Could you check a few things on this model? Use its own coordinates, in mm. A direction names the side the tool comes from. Coordinates: 2 decimals unless noted, no trailing zeros. Loops run counter-clockwise (first coordinate to the right, second up) from the corner with the lowest first, then second, coordinate; pieces in that order, holes last. Notation, with made-up numbers: M -37,31.25 L 2,31.25 A23 ccw 2,66.25 Z; hole C -9.5,32 d4. An arc over 180 degrees is marked long. Write each question's results on one line, items separated by ' | '.
Autodesk Fusion 360 part; units mm, degrees
sketch "Sketch1" plane through (0, 0, 0) normal (1, 0, 0) x (0, 1, 0)
  line L0 (0, 0) -> (0, 45)
  line L1 (0, 0) -> (0, -45)
  line L2 (0, 45) -> (37.5, 45)
  line L3 (0, 45) -> (-37.5, 45)
  line L4 (0, -45) -> (37.5, -45)
  line L5 (0, -45) -> (-37.5, -45)
  arc A0 (37.5, -45) -> (37.5, 45) centre (-79.119, 0) ccw
  arc A1 (-37.5, 45) -> (-37.5, -45) centre (79.119, 0) ccw
  dimension "d1" = 45
  dimension "d2" = 45
  dimension "d3" = 37.5
  dimension "d4" = 37.5
  dimension "d6" = 125
extrude "Extrude1" add sketch "Sketch1" along normal blind 100
sketch "Sketch2" plane through (0, 0, 0) normal (1, 0, 0) x (0, 1, 0)
extrude "Extrude2" add 1 faces at (100, 14.2806, 15.2642) along direction (1, 0, 0) blind 35 draft -15
sketch "Sketch3" plane through (0, 0, 0) normal (-1, 0, 0) x (0, -1, 0)
  line L0 (37.5, 45) -> (-37.5, 45)
  arc A0 (-37.5, 45) -> (-37.5, -45) centre (79.119, 0) ccw
  line L1 (-37.5, -45) -> (37.5, -45)
  arc A1 (37.5, -45) -> (37.5, 45) centre (-79.119, 0) ccw
sketch "Sketch4" plane through (135, 0, 0) normal (1, 0, 0) x (0, 1, 0)
  line L0 (30.8786, 35.6218) -> (-30.8786, 35.6218)
  arc A0 (-30.8786, 35.6218) -> (-30.8786, -35.6218) centre (79.119, 0) ccw
  line L1 (-30.8786, -35.6218) -> (30.8786, -35.6218)
  arc A1 (30.8786, -35.6218) -> (30.8786, 35.6218) centre (-79.119, 0) ccw
  circle A2 centre (0, 0) radius 34.5
  dimension "d11" = 69
extrude "Extrude3" add sketch "Sketch4" along normal blind 10 contours A2
sketch "Sketch5" plane through (145, 0, 0) normal (1, 0, 0) x (0, 1, 0)
  circle A0 centre (0, 0) radius 34.5
  circle A1 centre (0, 0) radius 31
  dimension "d14" = 62
extrude "Extrude4" add sketch "Sketch5" along normal blind 30 contours A1
sketch "Sketch6" plane through (175, 0, 0) normal (1, 0, 0) x (0, 1, 0)
  circle A0 centre (0, 0) radius 31
  line L0 (0, 0) -> (27, 0)
  circle A1 centre (27, 0) radius 2.5
  circle A2 centre (27, 0) radius 1.5
  dimension "d17" = 27
  dimension "d18" = 5
  dimension "d19" = -1
extrude "Extrude5" add sketch "Sketch6" along normal blind 1 contours A1
sketch "Sketch7" plane through (175, 0, 0) normal (1, 0, 0) x (0, 1, 0)
  circle A0 centre (0, 0) radius 31
  circle A1 centre (27, 0) radius 2.5
sketch "Sketch8" plane through (175, 0, 0) normal (1, 0, 0) x (0, 1, 0)
sketch "Sketch9" plane through (175, 0, 0) normal (1, 0, 0) x (0, 1, 0)
pattern_circular "C-Pattern1" count 12 over 360 about axis through (1.75, 0, 0) along (1, 0, 0) of "Extrude5"
sketch "Sketch10" plane through (175, 0, 0) normal (1, 0, 0) x (0, 1, 0)
  line L0 (0, 0) -> (16, 0)
  line L1 (16, 0) -> (16, 17)
  line L2 (16, 0) -> (16, -17)
  line L3 (0, 0) -> (0, -10)
  line L4 (-16, 0) -> (-16, 17)
  line L5 (-16, 0) -> (-16, -17)
  arc A0 (16, 17) -> (-16, 17) centre (0, 1.9003) ccw
  arc A1 (-16, -17) -> (16, -17) centre (0, -1.9003) ccw
  dimension "d24" = 16
  dimension "d25" = 17
  dimension "d26" = 17
  dimension "d27" = 22
  dimension "d28" = 22
extrude "Extrude6" add sketch "Sketch10" along normal blind 100
sketch "Sketch11" plane through (275, 0, 0) normal (1, 0, 0) x (0, 1, 0)
  line L0 (-16, 17) -> (-16, -17)
  arc A0 (-16, -17) -> (16, -17) centre (0, -1.9003) ccw
  line L1 (16, -17) -> (16, 17)
  arc A1 (16, 17) -> (-16, 17) centre (0, 1.9003) ccw
  circle A2 centre (0, 0) radius 30.9877
extrude "Extrude7" add sketch "Sketch11" along normal blind 10 contours L0 A0 L1 A1 | A2
sketch "Sketch12" plane through (285, 0, 0) normal (1, 0, 0) x (0, 1, 0)
  circle A0 centre (0, 0) radius 30.9877
  circle A1 centre (0, 0) radius 29.9877
  dimension "d33" = -1
extrude "Extrude8" add sketch "Sketch12" along normal blind 1 contours A1
extrude "Extrude9" add 1 faces at (286, 6.5805, -3.169) along direction (1, 0, 0) blind 10
sketch "Sketch13" plane through (0, 0, 0) normal (0, 1, 0) x (1, 0, 0)
ref_plane "WorkPlane1" through (0, -37.5, 45) normal (0, -1, 0) x (1, 0, 0)
sketch "Sketch14" plane through (0, -37.5, 0) normal (0, -1, 0) x (-1, 0, 0)
  circle A0 centre (-50, 45) radius 42.5
  dimension "d38" = 85
extrude "Extrude10" add sketch "Sketch14" along normal mid plane 21
sketch "Sketch15" plane through (0, -27, 0) normal (0, 1, 0) x (-1, 0, 0)
  line L0 (-7.5, -45) -> (-92.5, -45)
  arc A0 (-92.5, -45) -> (-7.5, -45) centre (-50, -45) ccw
  line L1 (-50, -45) -> (-50, -75)
  line L2 (-70, -45) -> (-70, -75)
  line L3 (-30, -45) -> (-30, -75)
  arc A1 (-70, -75) -> (-30, -75) centre (-50, -60) ccw
  line L4 (-70, -45) -> (-50, -45)
  line L5 (-50, -45) -> (-30, -45)
  line L6 (-70, -75) -> (-50, -75)
  line L7 (-30, -75) -> (-50, -75)
  dimension "d41" = 30
  dimension "d42" = 20
  dimension "d43" = -20
  dimension "d44" = 25
extrude "Extrude11" add sketch "Sketch15" along normal blind 35 contours L0 L1 L3 L5 L7 | L0 L1 L2 L4 L6 | A1 L6 L7
sketch "Sketch16" plane through (70, 0, 0) normal (1, 0, 0) x (0, 1, 0)
  line L0 (-27, -45) -> (-27, -75)
  line L1 (-27, -75) -> (8, -75)
  line L2 (8, -75) -> (8, -45)
  line L3 (8, -45) -> (-27, -45)
  line L4 (8, -45) -> (33, -45)
  line L5 (8, -45) -> (8, -87)
  arc A0 (8, -87) -> (33, -45) centre (-21.8393, -40.7981) ccw
  dimension "d47" = 25
  dimension "d48" = 42
  dimension "d49" = 55
extrude "Extrude12" add sketch "Sketch16" against normal blind 40 contours L2 L4 L5 A0
sketch "Sketch17" plane through (0, 8, 0) normal (0, -1, 0) x (1, 0, 0)
  arc A0 (30, -75) -> (70, -75) centre (50, -60) ccw
  line L0 (30, -75) -> (30, -87)
  line L1 (30, -87) -> (70, -87)
  line L2 (70, -87) -> (70, -75)
extrude "Extrude13" cut sketch "Sketch17" against normal blind 40
sketch "Sketch18" plane through (296, 0, 0) normal (1, 0, 0) x (0, 1, 0)
  circle A0 centre (0, 0) radius 29.9877
  circle A1 centre (0, 0) radius 15
  dimension "d54" = 30
extrude "Extrude14" cut sketch "Sketch18" against normal blind 20 contours A1
sketch "Sketch19" plane through (0, -48, 0) normal (0, -1, 0) x (1, 0, 0)
  circle A0 centre (50, -45) radius 42.5
  circle A1 centre (50, -45) radius 15
  dimension "d57" = 30
extrude "Extrude15" cut sketch "Sketch19" against normal blind 19 contours A1
sketch "Sketch20" plane through (0, -48, 0) normal (0, -1, 0) x (1, 0, 0)
  circle A0 centre (50, -45) radius 15
  circle A1 centre (50, -45) radius 42.5
equation "d39 = ( 21 / 2 ) * 1 mm"
(1) Imagine slicing it at A-A, the plane x = 50. List the corners of the cut face in (y, z) for me.
Reported:
outline: M -48,-87.5 L -27,-87.5 L -27,-85 L 10.89,-85 A55 ccw 33,-45 L 37.5,-45 A125 ccw 37.5,45 L -37.5,45 A125 ccw -45.86,-2.5 L -48,-2.5 L -48,-30 L -29,-30 L -29,-60 L -48,-60 Z
(2) Please list where these lines run through material, in increasing order: probe 1 along Y at (x, z) = (175.45, -13.5); probe 2 along X at (y, z) = (22, -16); probe 3 along X at (y, z) = (19.5, 26.5). Write a range as from..to.
Reported:
probe 1: y = -25.88..-24.88, -21.88..-20.88, -16..16, 20.88..21.88, 24.88..25.88 | probe 2: x = 0..175, 275..296 | probe 3: x = 0..145
(3) Will these pins go through, and if not, where does the flat tip stop? P1, Ø10, axis at x = 202, z = -10, coming from the +Y side; P2, Ø15, axis at y = -6.5, z = -56, coming from the -X side; P3, Ø12, axis at x = 107, y = -28.5, coming from the -Z side.
Reported:
P1: stops at y = 16 | P2: stops at x = 30 | P3: stops at z = -44.73
(4) Imagine slicing it at C-C, the plane x = 266. List the corners of the cut face in (y, z) for me.
Reported:
outline: M -16,-17 A22 ccw 16,-17 L 16,17 A22 ccw -16,17 Z
(5) Which directions (+Z, -Z, +X, -X, +Y, -Y) give clear straight access to the entire face, cutting with the end or side of a thin tool? Please do faces 1 (the flat face through (175, -16.2, 0.1)), 2 (the cylindrical face through (50, -9, -85)), 3 (the cylindrical face through (139.93, 32.907, -10.363)).
Reported:
face 1: none | face 2: -Z, +Y | face 3: +X
(6) Imagine slicing it at B-B, the plane z = -69. List the corners of the cut face in (x, y) for me, and give its area (3 significant figures).
Reported:
outline: M 14.93,-48 L 85.07,-48 L 85.07,-27 L 70,-27 L 70,25.38 L 30,25.38 L 30,-27 L 14.93,-27 Z | area: 3,570 mm2
(7) If we mould it in two halves opening along X, with no side actions, what happens to faces 4 (the flat face through (135, -5.6, 34.5)), 5 (the flat face through (51, -48, -27)), 6 (the cylindrical face through (224.3, 0.3, -23.9))? For each: released by +X, released by -X, zero draft, split by the parting line, or undercut.
Reported:
face 4: released by +X | face 5: zero draft | face 6: undercut
